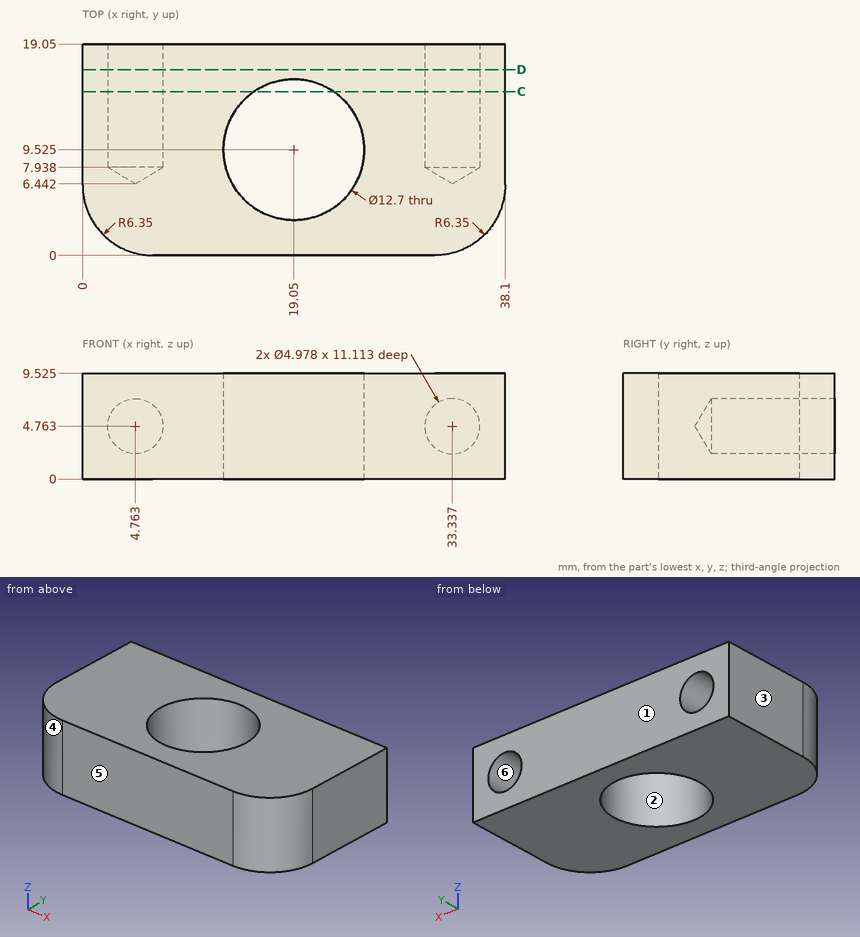
Verification items for this drawing (mm, ordinates from the low corner). A direction names the side the tool comes from. Give positions to 0.01 mm unless a question says otherwise; leave off trailing zeros. Loops run counter-clockwise (first coordinate to the right, second up) from the corner with the lowest first, then second, coordinate; pieces in that order, holes last. Notation, with made-up numbers: M -32.5,89.5 L 24.5,89.5 A19 cw 24.5,93.5 Z; hole C 10,60 d5. An arc over 180 degrees is marked long. Write item = value, one per line.
(1) Material ranges on line 1 (X direction, y = 10.25, z = 5) (1 decimal); line 2 (X direction, y = 18, z = 5.5) (1 decimal); line 3 (X direction, y = 13, z = 6.5) (1 decimal), recorded low to high. Write a range as [from, to].
Answer below:
line_1 = [0, 2.3], [7.2, 12.7], [25.4, 30.9], [35.8, 38.1]
line_2 = [0, 2.4], [7.1, 31], [35.7, 38.1]
line_3 = [0, 3], [6.5, 13.7], [24.4, 31.6], [35.1, 38.1]
(2) Sectioned sample at C-C, the plane y = 14.75. Record the cut outline in (x, z) (1 decimal), plus the area to 3 significant figures.
Answer below:
outline = M 0,0 L 15.4,0 L 15.4,9.5 L 0,9.5 Z; M 22.7,0 L 38.1,0 L 38.1,9.5 L 22.7,9.5 Z; hole C 4.8,4.8 d5; hole C 33.3,4.8 d5
area = 255 mm2
(3) Sectioned sample at D-D, the plane y = 16.75. Record the cut outline in (x, z) (1 decimal).
Answer below:
outline = M 0,0 L 38.1,0 L 38.1,9.5 L 0,9.5 Z; hole C 4.8,4.8 d5; hole C 33.3,4.8 d5
(4) Release check for a two-part mould opening along Y. For the marked faces 1, 2, 3 and 4 record: released by +Y, released by -Y, zero draft, split by the parting line, or undercut.
Answer below:
face_1 = released by +Y
face_2 = undercut
face_3 = zero draft
face_4 = released by -Y
(5) Tool access check on the marked faces 5 and 6. Record the directions out of +Z, -Z, +X, -X, +Y, -Y that give a thin tool (end or side, any length) a straight path to the whole face; none if there is none.
Answer below:
face_5 = +Z, -Z, +X, -X, -Y
face_6 = +Y
